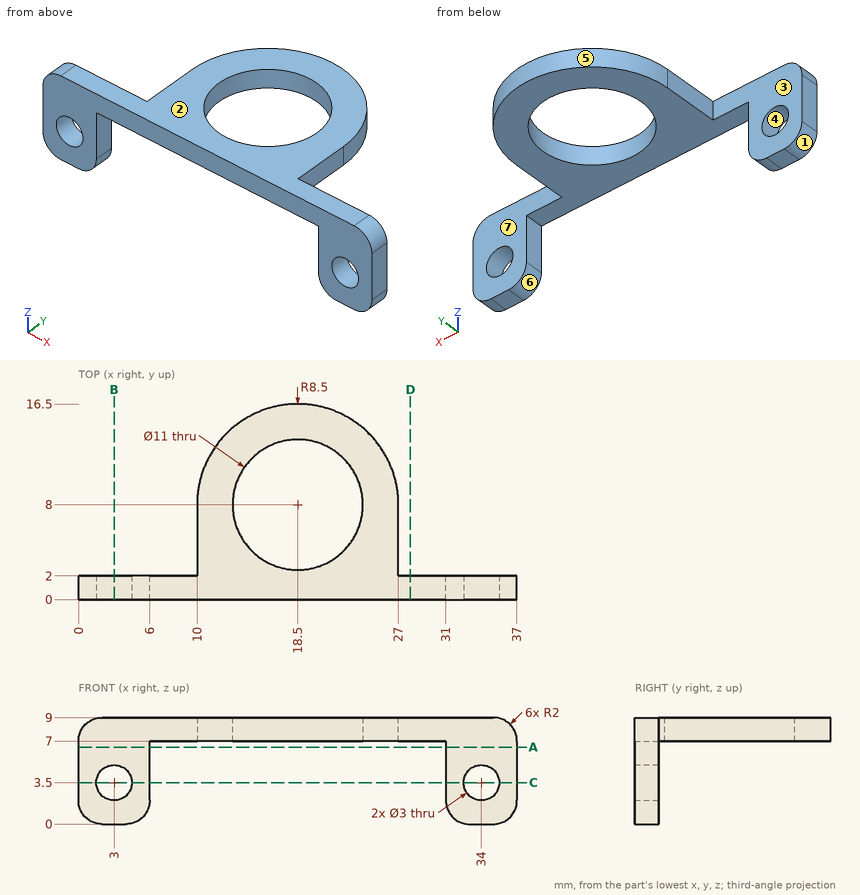
Answer from the drawing. Dimensions are ordinates in mm from the lowest x, y and z of the part. A direction names the side the tool comes from. Give positions to 0.01 mm unless a question says otherwise; leave off trailing zeros. Loops run counter-clockwise (first coordinate to the right, second up) from the corner with the lowest first, then second, coordinate; pieces in that order, holes last. Notation, with made-up numbers: (-18.5, 77.5) - (-8.5, 77.5) arc R16 ccw to (-8.5, 90.5) - close; hole circle Ø11 at (89, -30). An arc over 180 degrees is marked (long way). Answer as CSV lines item,"result". Start each with the question number.
Item 1: A cutting plane is placed at C-C on z = 3.5. Determine the outline of the cut face in (x, y), then the cut area to 3 significant figures.
Item 2: For the marked faces 5, 6 and 7, determine the directions among +Z, -Z, +X, -X, +Y, -Y from which every point of the face is accessible in a straight line to the end or side of a thin tool.
Item 3: A cutting plane is placed at D-D on x = 28. Determine the outline of the cut face in (y, z).
Item 4: Each of these flat-tipped pins is pushed along its axis until it touches: pin 1 (3.5 mm diameter, centred on x = 34, z = 3.5, fed in from +Y); pin 2 (0.6 mm diameter, centred on y = 6, z = 8.5, fed in from -X); pin 3 (5 mm diameter, centred on y = 14, z = 8, fed in from +X). Where does it stop, or does it pass through?
Item 5: A cutting plane is placed at A-A on z = 6.5. Determine the outline of the cut face in (x, y).
Item 6: A cutting plane is placed at B-B on x = 3. Determine the outline of the cut face in (y, z), then the cut area to 3 significant figures.
Item 7: The mould has two halves that part along Z. Classify the marked faces 1, 2, 3 and 4: +Z half, -Z half, draft (parallel to the pull), parting line (faces both ways), or undercut.
Item 8: Find the intervals of material crossed by line 1 (X direction, y = 1.5, z = 3.5); line 2 (Z direction, x = 25.5, y = 5.5); line 3 (Y direction, x = 34, z = 5.25), in increasing order. Write a range as from..to.
Found:
1,outline,"(0, 0) - (1.5, 0) - (1.5, 2) - (0, 2) - close; (4.5, 0) - (6, 0) - (6, 2) - (4.5, 2) - close; (31, 0) - (32.5, 0) - (32.5, 2) - (31, 2) - close; (35.5, 0) - (37, 0) - (37, 2) - (35.5, 2) - close"
1,area,"12.0 mm^2"
2,face 5,"+Z, -Z, +Y"
2,face 6,"-Z, +Y, -Y"
2,face 7,"+Z, -Z, +X, +Y"
3,outline,"(0, 7) - (2, 7) - (2, 9) - (0, 9) - close"
4,pin 1,"stops at y = 2"
4,pin 2,"stops at x = 10"
4,pin 3,"stops at x = 26.25"
5,outline,"(0, 0) - (6, 0) - (6, 2) - (0, 2) - close; (31, 0) - (37, 0) - (37, 2) - (31, 2) - close"
6,outline,"(0, 0) - (2, 0) - (2, 2) - (0, 2) - close; (0, 5) - (2, 5) - (2, 9) - (0, 9) - close"
6,area,"12.0 mm^2"
7,face 1,"-Z half"
7,face 2,"+Z half"
7,face 3,"draft"
7,face 4,"undercut"
8,line 1,"x = 0..1.5, 4.5..6, 31..32.5, 35.5..37"
8,line 2,"z = 7..9"
8,line 3,"y = 0..2"
